Part print with two shaded views. Sizes in mm from the minimum x, y, z corner. A direction names the side the tool comes from. Round coordinates to 2 decimals unless told otherwise and drop trailing zeros. Loops run counter-clockwise (first coordinate to the right, second up) from the corner with the lowest first, then second, coordinate; pieces in that order, holes last. Notation, with made-up numbers: M 70,38 L 91,38 A14 ccw 91,46 Z; hole C 40.5,-37 d5. An arc over 180 degrees is marked long. Use a Markdown table: item, result. Add a question column.
Item 1: Pin check, flat tips, straight feed: P1, Ø16, axis at x = 46, z = 107, coming from the -Y side; P2, Ø2, axis at x = 44, y = 0.5, coming from the +Z side. Stop position of each tip, or through.
Item 2: Saw through at A-A on x = 70. Write the cut outline in (y, z).
Item 3: Saw through at C-C on z = 85. Write the cut outline in (x, y).
Item 4: Saw through at B-B on y = 0.9. Write the cut outline in (x, z).
Item 5: Tool access for the marked faces 1 and 2: list every direction of +Z, -Z, +X, -X, +Y, -Y with a clear straight run to the whole face (end or side of a thin tool).
Item 6: Saw through at D-D on x = 42. Write the cut outline in (y, z).
Item 7: Wall check: L1, parallel to X at y = 2.75, z = 10; L2, parallel to Z at x = 3, y = 2.35; L3, parallel to Z at x = 70, y = 0.95. Give the ranges that are in metal, low to high. Write a range as from..to.
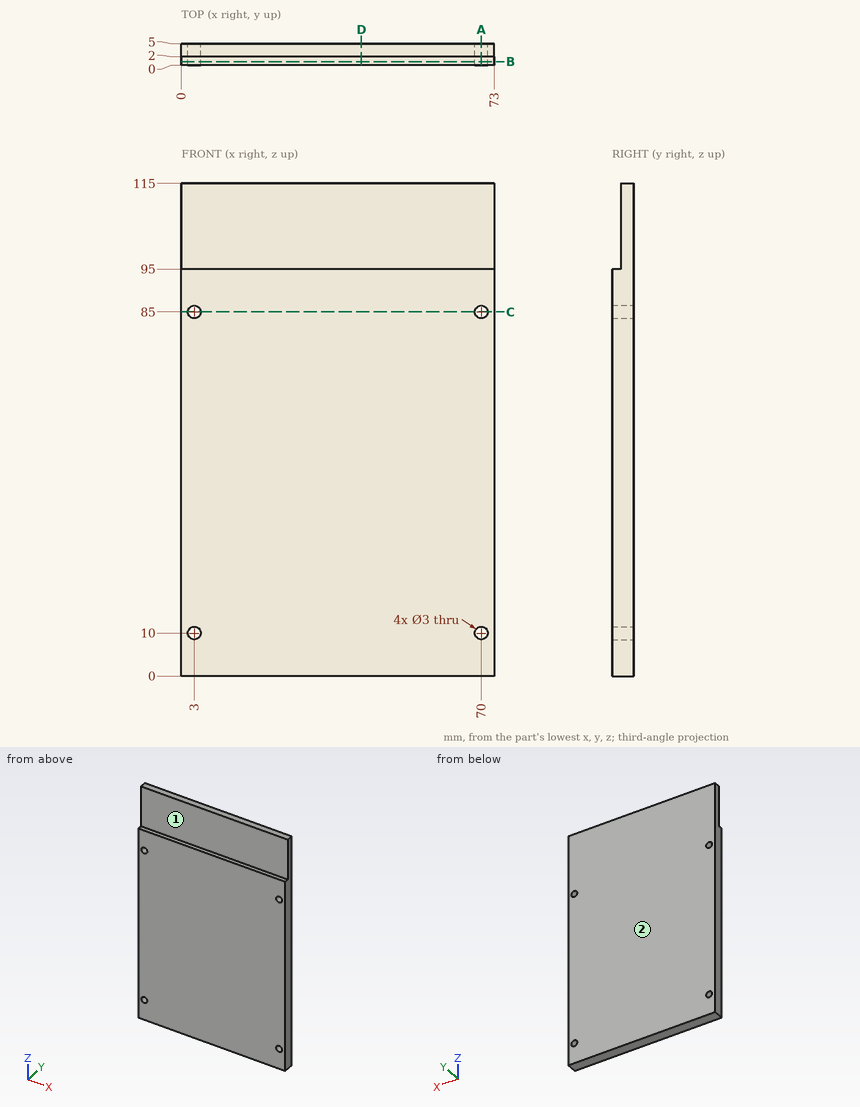
Entries:
| question | item | result |
|---|---|---|
| 1 | P1 | y = 2 |
| 1 | P2 | z = 95 |
| 2 | outline | M 0,0 L 5,0 L 5,8.5 L 0,8.5 Z; M 0,11.5 L 5,11.5 L 5,83.5 L 0,83.5 Z; M 0,86.5 L 5,86.5 L 5,115 L 2,115 L 2,95 L 0,95 Z |
| 3 | outline | M 0,0 L 1.5,0 L 1.5,5 L 0,5 Z; M 4.5,0 L 68.5,0 L 68.5,5 L 4.5,5 Z; M 71.5,0 L 73,0 L 73,5 L 71.5,5 Z |
| 4 | outline | M 0,0 L 73,0 L 73,95 L 0,95 Z; hole C 3,10 d3; hole C 3,85 d3; hole C 70,10 d3; hole C 70,85 d3 |
| 5 | face 1 | +Z, +X, -X, -Y |
| 5 | face 2 | +Z, -Z, +X, -X, +Y |
| 6 | outline | M 0,0 L 5,0 L 5,115 L 2,115 L 2,95 L 0,95 Z |
| 7 | L1 | 0..1.5, 4.5..68.5, 71.5..73 |
| 7 | L2 | 0..8.5, 11.5..83.5, 86.5..115 |
| 7 | L3 | 0..8.5, 11.5..83.5, 86.5..95 |
